```python
from build123d import *

# Parameters (mm, degrees)
SKETCH2_W           = 5
SKETCH2_H           = 5
BOSS_EXTRUDE1_DEPTH = 5
CUT_EXTRUDE1_DEPTH  = 2.5


with BuildPart() as part:
    # Sketch2 → Boss-Extrude1 (new body)
    with BuildSketch(Plane(origin=(0, 0, 0), x_dir=(1, 0, 0), z_dir=(0, 1, 0))):
        with BuildLine():
            Line((5, 0), (45, 0))
            ThreePointArc((45, 0), (48.535533906, -1.464466094), (50, -5))
            Line((50, -5), (50, -45))
            ThreePointArc((50, -45), (48.535533906, -48.535533906), (45, -50))
            Line((45, -50), (5, -50))
            ThreePointArc((5, -50), (1.464466094, -48.535533906), (0, -45))
            Line((0, -45), (0, -5))
            ThreePointArc((0, -5), (1.464466094, -1.464466094), (5, 0))
        make_face()
        with Locations((6.5, -25)):
            Rectangle(SKETCH2_W, SKETCH2_H, mode=Mode.SUBTRACT)
        with Locations((43.5, -25)):
            Rectangle(SKETCH2_W, SKETCH2_H, mode=Mode.SUBTRACT)
    extrude(amount=BOSS_EXTRUDE1_DEPTH)

    # Sketch4 → Cut-Extrude1 (cut)
    with BuildSketch(Plane(origin=(0, 5, 0), x_dir=(1, 0, 0), z_dir=(0, 1, 0))):
        with BuildLine():
            Line((23.299566157, -17.331191341), (14.010613466, -10.951334614))
            ThreePointArc((14.010613466, -10.951334614), (12.563442924, -10.574062008), (11.209455823, -11.209165249))
            ThreePointArc((11.209455823, -11.209165249), (10.574352582, -12.56315235), (10.951625187, -14.010322893))
            Line((10.951625187, -14.010322893), (17.331481915, -23.299275583))
            ThreePointArc((17.331481915, -23.299275583), (17.858572583, -24.997719905), (17.331481915, -26.696164227))
            Line((17.331481915, -26.696164227), (10.951625187, -35.985116918))
            ThreePointArc((10.951625187, -35.985116918), (10.574352582, -37.43228746), (11.209455823, -38.786274561))
            ThreePointArc((11.209455823, -38.786274561), (12.563442924, -39.421377802), (14.010613466, -39.044105197))
            Line((14.010613466, -39.044105197), (23.299566157, -32.664248469))
            ThreePointArc((23.299566157, -32.664248469), (24.998010479, -32.137157801), (26.696454801, -32.664248469))
            Line((26.696454801, -32.664248469), (35.985407491, -39.044105197))
            ThreePointArc((35.985407491, -39.044105197), (37.432578034, -39.421377802), (38.786565135, -38.786274561))
            ThreePointArc((38.786565135, -38.786274561), (39.421668376, -37.43228746), (39.04439577, -35.985116918))
            Line((39.04439577, -35.985116918), (32.664539043, -26.696164227))
            ThreePointArc((32.664539043, -26.696164227), (32.137448374, -24.997719905), (32.664539043, -23.299275583))
            Line((32.664539043, -23.299275583), (39.04439577, -14.010322893))
            ThreePointArc((39.04439577, -14.010322893), (39.421668376, -12.56315235), (38.786565135, -11.209165249))
            ThreePointArc((38.786565135, -11.209165249), (37.432578034, -10.574062008), (35.985407491, -10.951334614))
            Line((35.985407491, -10.951334614), (26.696454801, -17.331191341))
            ThreePointArc((26.696454801, -17.331191341), (24.998010479, -17.85828201), (23.299566157, -17.331191341))
        make_face()
    extrude(amount=-CUT_EXTRUDE1_DEPTH, mode=Mode.SUBTRACT)


solid = part.part
```
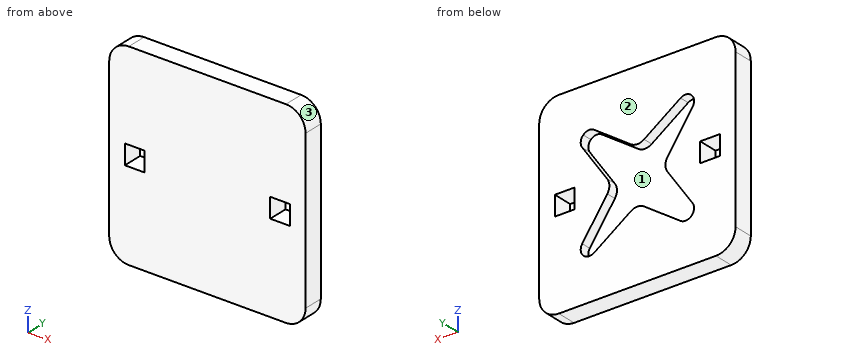
Can you work these out from the model? Positions are in its coordinate system, mm. Face numbers are marked on the shaded views. Coordinates: 2 decimals unless noted, no trailing zeros. Write each loop counter-clockwise with the first axis right and the second up, starting at its lowest first coordinate (ties: lowest second). Pieces come first, ordered by that corner, then holes. Notation, with made-up numbers: (37, 53.5) - (55, 53.5) arc R37 cw to (55, 91.5) - close; hole circle Ø6 at (-24.75, 61). An arc over 180 degrees is marked (long way). Return JSON: item names as keys, results as strings.
Q1. If we section it at D-D (z = 19): Please give me the cut outline in (x, y).
Computed values:
{"outline": "(0, 0) - (50, 0) - (50, 5) - (35.62, 5) - (35.62, 2.5) - (14.38, 2.5) - (14.38, 5) - (0, 5) - close"}
Q2. If we section it at A-A (z = 24): Please give me the cut outline in (x, y), then the cut area to 3 significant figures.
Computed values:
{"outline": "(0, 0) - (4, 0) - (4, 5) - (0, 5) - close; (9, 0) - (41, 0) - (41, 5) - (32.31, 5) - (32.31, 2.5) - (17.69, 2.5) - (17.69, 5) - (9, 5) - close; (46, 0) - (50, 0) - (50, 5) - (46, 5) - close", "area": "163 mm2"}
Q3. If we section it at C-C (x = 38): Please give me the cut outline in (y, z).
Computed values:
{"outline": "(0, 0) - (5, 0) - (5, 10.7) - (2.5, 10.7) - (2.5, 15.53) - (5, 15.53) - (5, 34.46) - (2.5, 34.46) - (2.5, 39.29) - (5, 39.29) - (5, 50) - (0, 50) - close"}
Q4. I'm going to push a flat-ended pin straight in: pin 1 Ø1 at (x, z) = (15, 12.5) entering from +Y. Where does the tip first touch, or does it pass through?
Computed values:
{"pin 1": "stops at y = 2.5"}
Q5. Thinking about a two-plate mould opening in Z: for the marked faces 1, 2 and 3, which applies, +Z half, -Z half, draft (parallel to the pull), parting line (faces both ways), or undercut?
Computed values:
{"face 1": "undercut", "face 2": "draft", "face 3": "+Z half"}
Q6. If we section it at B-B (y = 0.9): Please give me the cut outline in (x, z), then the cut area to 3 significant figures.
Computed values:
{"outline": "(0, 5) arc R5 ccw to (5, 0) - (45, 0) arc R5 ccw to (50, 5) - (50, 45) arc R5 ccw to (45, 50) - (5, 50) arc R5 ccw to (0, 45) - close; hole (4, 22.5) - (9, 22.5) - (9, 27.5) - (4, 27.5) - close; hole (41, 22.5) - (46, 22.5) - (46, 27.5) - (41, 27.5) - close", "area": "2,430 mm2"}
Q7. Please list where these lines run through material, in increasing order: L1, parallel to Z at x = 16.5, y = 3.05; L2, parallel to X at y = 3.7, z = 24; L3, parallel to X at y = 3.15, z = 17 (3 decimals). Write a range as from..to.
Computed values:
{"L1": "z = 0..12.66, 22.09..27.91, 37.33..50", "L2": "x = 0..4, 9..17.69, 32.31..41, 46..50", "L3": "x = 0..13.005, 22.817..27.179, 36.991..50"}
